Here's how the part is built. I have some questions about the finished solid (model axes, mm). A direction names the side the tool comes from. Round coordinates to 2 decimals unless told otherwise and drop trailing zeros. Write each loop counter-clockwise with the first axis right and the second up, starting at its lowest first coordinate (ties: lowest second). Pieces come first, ordered by that corner, then holes. Notation, with made-up numbers: M -4,-9 L 19,-9 A19 cw 19,24 Z; hole C 68,7 d5. An arc over 180 degrees is marked long. Write item = value, one per line. Start each with the question number.
(1) I want a section at C-C (z = 0.6). Give the number of separate pieces and of enclosed holes in the cut face, and give its area (3 significant figures).
(2) Will these pins go through, and if not, where does the flat tip stop? pin 1 Ø0.9 at (y, z) = (10, 2) entering from -X; pin 2 Ø0.5 at (x, z) = (1.5, 1) entering from -Y; pin 3 Ø1 at (y, z) = (22, 0.5) entering from -X (3 decimals); pin 4 Ø2.5 at (x, y) = (28.275, 21.96) entering from +Z.
(3) I want a section at B-B (x = 16.5). List the corners of the cut face in (y, z) for me.
(4) I want a section at A-A (y = -5.04). List the corners of the cut face in (x, z) for me (3 decimals).
(5) I need wall thicknesses on line 1 along X through (y, z) = (2.5, 0.85); line 2 along X through (y, z) = (10.5, 0.85); line 3 along X through (y, z) = (21.96, 1.85) (3 decimals). Which ranges of each line are inside material? Lowest first, please.
(6) If we mould it in two halves opening along Y, with no side actions, what happens to faces 6 (the cylindrical face through (-0.05, 16.99, 1.48)), 7 (the cylindrical face through (29.189, 23.393, 1.479)), 8 (the flat face through (15, 16, 3))? For each: released by +Y, released by -Y, zero draft, split by the parting line, or undercut.
(7) On a 3-axis mill with a long thin cutter (end or side, diameter ignored), from which of +Z, -Z, +X, -X, +Y, -Y can I reach the whole of each face in a straight line? I mean faces 1 (the cylindrical face through (-0.07, -0.05, 1.48)), 2 (the flat face through (30.275, 18, 1)), 3 (the cylindrical face through (2.378, 17.555, 1.479)), 4 (the flat face through (1.5, 9, 1)), 5 (the flat face through (32.8, 8, 1)). Say none if no direction works.
(8) I want a section at D-D (y = 17). List the corners of the cut face in (x, z) for me.
```python
from build123d import *

# Parameters (mm, degrees)
PCB_EDGE_SUPPORT_DEPTH       = 3
SKETCH_2_R                   = 3
PCB_SCREW_LANDS_DEPTH        = 3
SKETCH_3_W                   = 4
SKETCH_3_H                   = 7.04
FLOATING_MOUNT_BRIDGES_DEPTH = 3
SKETCH_4_R                   = 4
FLOATING_MOUNT_EARS_DEPTH    = 3
SKETCH_5_R                   = 1.15
PCB_M2_CLEARANCE_DEPTH       = 4
SKETCH_6_R                   = 1.7
M2_ADJUSTMENT_0P7_DEPTH      = 4


with BuildPart() as part:
    # 草图1 → PCB_edge_support (new body)
    with BuildSketch(Plane.XY):
        with BuildLine():
            Line((1, -0.5), (31.3, -0.5))
            ThreePointArc((31.3, -0.5), (32.360660172, -0.060660172), (32.8, 1))
            Line((32.8, 1), (32.8, 15.92))
            ThreePointArc((32.8, 15.92), (32.360660172, 16.980660172), (31.3, 17.42))
            Line((31.3, 17.42), (1, 17.42))
            ThreePointArc((1, 17.42), (-0.060660172, 16.980660172), (-0.5, 15.92))
            Line((-0.5, 15.92), (-0.5, 1))
            ThreePointArc((-0.5, 1), (-0.060660172, -0.060660172), (1, -0.5))
        make_face()
        with BuildLine():
            Line((2.5, 1.5), (29.8, 1.5))
            ThreePointArc((29.8, 1.5), (30.507106781, 1.792893219), (30.8, 2.5))
            Line((30.8, 2.5), (30.8, 14.42))
            ThreePointArc((30.8, 14.42), (30.507106781, 15.127106781), (29.8, 15.42))
            Line((29.8, 15.42), (2.5, 15.42))
            ThreePointArc((2.5, 15.42), (1.792893219, 15.127106781), (1.5, 14.42))
            Line((1.5, 14.42), (1.5, 2.5))
            ThreePointArc((1.5, 2.5), (1.792893219, 1.792893219), (2.5, 1.5))
        make_face(mode=Mode.SUBTRACT)
    extrude(amount=PCB_EDGE_SUPPORT_DEPTH)

    # 草图2 → PCB_screw_lands (add)
    with BuildSketch(Plane.XY):
        with Locations((2.365, 2.365)):
            Circle(SKETCH_2_R)
        with Locations((2.365, 14.555)):
            Circle(SKETCH_2_R)
    extrude(amount=PCB_SCREW_LANDS_DEPTH)

    # 草图3 → Floating_mount_bridges (add)
    with BuildSketch(Plane.XY):
        with Locations((4.275, -1.52)):
            Rectangle(SKETCH_3_W, SKETCH_3_H)
        with Locations((28.275, 18.44)):
            Rectangle(SKETCH_3_W, SKETCH_3_H)
    extrude(amount=FLOATING_MOUNT_BRIDGES_DEPTH)

    # 草图4 → Floating_mount_ears (add)
    with BuildSketch(Plane.XY):
        with Locations((4.275, -5.04)):
            Circle(SKETCH_4_R)
        with Locations((28.275, 21.96)):
            Circle(SKETCH_4_R)
    extrude(amount=FLOATING_MOUNT_EARS_DEPTH)

    # 草图5 → PCB_M2_clearance (cut)
    with BuildSketch(Plane.XY):
        with Locations((2.365, 2.365)):
            Circle(SKETCH_5_R)
        with Locations((2.365, 14.555)):
            Circle(SKETCH_5_R)
    extrude(amount=PCB_M2_CLEARANCE_DEPTH, mode=Mode.SUBTRACT)

    # 草图6 → M2_adjustment_0p7 (cut)
    with BuildSketch(Plane.XY):
        with Locations((4.275, -5.04)):
            Circle(SKETCH_6_R)
        with Locations((28.275, 21.96)):
            Circle(SKETCH_6_R)
    extrude(amount=M2_ADJUSTMENT_0P7_DEPTH, mode=Mode.SUBTRACT)


solid = part.part
```
Returned:
q1.separate_pieces = 1
q1.enclosed_holes = 5
q1.area = 296 mm²
q2.pin_1 = -0.5
q2.pin_2 = -8.14
q2.pin_3 = 24.275
q2.pin_4 = through
q3.outline = M -0.5,0 L 1.5,0 L 1.5,3 L -0.5,3 Z; M 15.42,0 L 17.42,0 L 17.42,3 L 15.42,3 Z
q4.outline = M 0.275,0 L 2.575,0 L 2.575,3 L 0.275,3 Z; M 5.975,0 L 8.275,0 L 8.275,3 L 5.975,3 Z
q5.line_1 = -0.63 to 1.22, 3.51 to 5.36, 30.8 to 32.8
q5.line_2 = -0.5 to 1.5, 30.8 to 32.8
q5.line_3 = 24.275 to 26.575, 29.975 to 32.275
q6.face_6 = released by +Y
q6.face_7 = undercut
q6.face_8 = zero draft
q7.face_1 = +Z, -Z, -X
q7.face_2 = +Z, -Z, +X
q7.face_3 = +Z, -Z, +Y
q7.face_4 = +Z, -Z
q7.face_5 = +Z, -Z, +X, +Y, -Y
q8.outline = M -0.04,0 L 32.34,0 L 32.34,3 L -0.04,3 Z
